Could you check a few things on this model? Use its own coordinates, in mm. Face numbers are marked on the shaded views. A direction names the side the tool comes from. Coordinates: 2 decimals unless noted, no trailing zeros. Loops run counter-clockwise (first coordinate to the right, second up) from the corner with the lowest first, then second, coordinate; pieces in that order, holes last.
Autodesk Inventor part; units mm, degrees
ref_plane "YZ Plane" through (0, 0, 0) normal (1, 0, 0) x (0, 1, 0)
ref_plane "XZ Plane" through (0, 0, 0) normal (0, 1, 0) x (-1, 0, 0)
ref_plane "XY Plane" through (0, 0, 0) normal (0, 0, 1) x (1, 0, 0)
sketch "Sketch1" plane through (0, 0, 0) normal (0, 1, 0) x (-1, 0, 0)
  line L0 (-21, -21) -> (21, -21)
  line L1 (21, -21) -> (21, 21)
  line L2 (21, 21) -> (-21, 21)
  line L3 (-21, 21) -> (-21, -21)
  line L4 (-21, -21) -> (21, 21) construction
  line L5 (21, -21) -> (-21, 21) construction
  point P0 (0, 0)
  dimension "d0" = 42
  dimension "d1" = 42
extrude "Extrusion1" add sketch "Sketch1" along normal blind 9
chamfer "Chamfer1" distance 6 angle 45 4 edges at (21, 4.5, -21) (-21, 4.5, -21) (-21, 4.5, 21) (21, 4.5, 21)
sketch "Sketch2" plane through (0, 9, 0) normal (0, 1, 0) x (1, 0, 0)
  point P0 (0, 0)
sketch "Sketch3" plane through (0, 0, 0) normal (0, -1, 0) x (1, 0, 0)
  circle A0 centre (0, 0) radius 5
  dimension "d7" = 10
extrude "Extrusion2" cut sketch "Sketch3" against normal up to surface (9 mm away)
sketch "Sketch4" plane through (0, 9, 0) normal (0, 1, 0) x (1, 0, 0)
  circle A0 centre (-15.5, -15.5) radius 1.5
  line L0 (-15, -21) -> (15, -21)
  line L1 (-21, 15) -> (-21, -15)
  point P0 (0, 0)
  dimension "d10" = 3
  dimension "d11" = 5.5
  dimension "d12" = 5.5
extrude "Extrusion3" cut sketch "Sketch4" against normal up to surface (9 mm away)
mirror "Mirror1" about plane through (0, 0, 0) normal (1, 0, 0) of "Extrusion3"
mirror "Mirror2" about plane through (0, 0, 0) normal (0, 0, 1) of "Extrusion3", "Mirror1"
sketch "Sketch6" plane through (0, 0, 0) normal (0, -1, 0) x (1, 0, 0)
  circle A0 centre (15.5, -15.5) radius 1.5
  circle A1 centre (-15.5, -15.5) radius 1.5
  circle A2 centre (15.5, 15.5) radius 1.5
  circle A3 centre (-15.5, 15.5) radius 1.5
  circle A4 centre (0, 0) radius 5
  line L0 (15, 21) -> (21, 15)
  line L1 (-15, 21) -> (15, 21)
  line L2 (-21, 15) -> (-15, 21)
  line L3 (-21, -15) -> (-21, 15)
  line L4 (-15, -21) -> (-21, -15)
  line L5 (15, -21) -> (-15, -21)
  line L6 (21, -15) -> (15, -21)
  line L7 (21, 15) -> (21, -15)
  line L8 (8, -21) -> (-8, -21)
  line L9 (-8, -21) -> (-8, -25)
  line L10 (-8, -25) -> (8, -25)
  line L11 (8, -25) -> (8, -21)
  dimension "d20" = 16
  dimension "d21" = 8
  dimension "d24" = 4
extrude "Extrusion5" add sketch "Sketch6" against normal blind 4 contours L11 L10 L9 L5
fillet "Fillet1" radius 0.5 2 edges at (8, 2, -25) (-8, 2, -25)
sketch "Sketch7" plane through (15, 9, -21) normal (0, 0, -1) x (-1, 0, 0)
  line L0 (23, -5) -> (23, -9)
  line L1 (23, -9) -> (30, -9)
  line L2 (30, 0) -> (30, -9)
  line L3 (0, 0) -> (30, 0)
  line L4 (0, -9) -> (0, 0)
  line L5 (0, -9) -> (7, -9)
  line L6 (7, -9) -> (7, -5)
  line L7 (7, -5) -> (23, -5)
  line L8 (7, -5) -> (23, -5)
  line L9 (23, -5) -> (23, 0)
  line L10 (23, 0) -> (7, 0)
  line L11 (7, 0) -> (7, -5)
  point P0 (15, -9)
extrude "Extrusion6" cut sketch "Sketch7" against normal blind 10 contours L7 L11 L3 L9
sketch "Sketch8" plane through (15, 9, -11) normal (0, 0, -1) x (-1, 0, 0)
  line L0 (23, -5) -> (7, -5)
  line L1 (23, 0) -> (23, -5)
  line L2 (7, 0) -> (23, 0)
  line L3 (7, -5) -> (7, 0)
  line L4 (23, 0) -> (23, -5)
  line L5 (7, -4.3) -> (23, -4.3)
  line L6 (23, -4.3) -> (23, -4.8)
  line L7 (23, -4.8) -> (7, -4.8)
  line L8 (7, -4.8) -> (7, -4.3)
  point P0 (15, -9)
  dimension "d28" = 0.5
  dimension "d29" = 0.2
extrude "Extrusion7" add sketch "Sketch8" along normal blind 15 contours L7 L3 L5 L1
sketch "Sketch9" plane through (15, 9, -11) normal (0, 0, -1) x (-1, 0, 0)
  point P0 (15, -9)
sketch "Sketch10" plane through (0, 0, 0) normal (0, -1, 0) x (1, 0, 0)
  circle A0 centre (15.5, 15.5) radius 1.5
  circle A1 centre (15.5, 15.5) radius 3
  point P0 (0, 0)
  dimension "d32" = 6
extrude "Extrusion8" cut sketch "Sketch10" against normal blind 3
mirror "Mirror3" about plane through (0, 0, 0) normal (1, 0, 0) of "Extrusion8"
mirror "Mirror4" about plane through (0, 0, 0) normal (0, 0, 1) of "Extrusion8", "Mirror3"
equation "\"d12\" = d11"
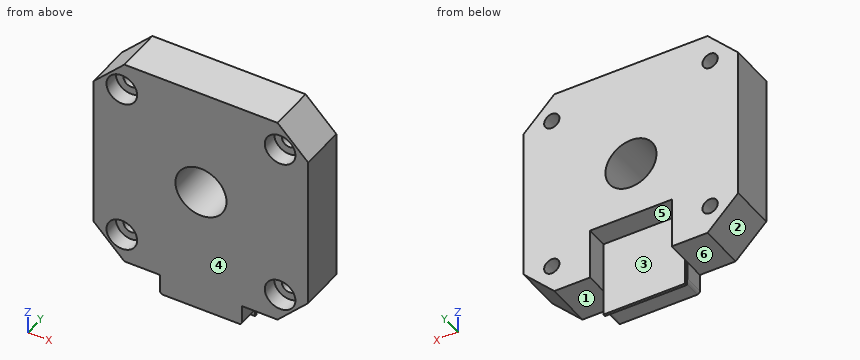
(1) Imagine slicing it at B-B, the plane x = 0. Write out the boundary of the cut face in (y, z).
Answers:
outline: (0, -25) - (4, -25) - (4, -11) - (4.2, -11) - (4.2, -26) - (4.7, -26) - (4.7, -11) - (9, -11) - (9, -5) - (0, -5) - close; (0, 5) - (9, 5) - (9, 21) - (0, 21) - close
(2) Imagine slicing it at A-A, the plane z = 0. Write out the boundary of the cut face in (x, y).
Answers:
outline: (-21, 0) - (-5, 0) - (-5, 9) - (-21, 9) - close; (5, 0) - (21, 0) - (21, 9) - (5, 9) - close
(3) Imagine slicing it at C-C, the plane y = 1. Write out the boundary of the cut face in (x, z), and give its area (3 significant figures).
Answers:
outline: (-21, -15) - (-15, -21) - (-8, -21) - (-8, -24.5) arc R0.5 ccw to (-7.5, -25) - (7.5, -25) arc R0.5 ccw to (8, -24.5) - (8, -21) - (15, -21) - (21, -15) - (21, 15) - (15, 21) - (-15, 21) - (-21, 15) - close; hole circle Ø6 at (-15.5, -15.5); hole circle Ø6 at (-15.5, 15.5); hole circle Ø10 at (0, 0); hole circle Ø6 at (15.5, -15.5); hole circle Ø6 at (15.5, 15.5)
area: 1,560 mm2
(4) Which directions (+Z, -Z, +X, -X, +Y, -Y) give clear straight access to the entire face, cutting with the end or side of a thin tool? Please do the marked faces 4, 5 and 6.
Answers:
face 4: +Z, -Z, +X, -X, -Y
face 5: -Z, +Y
face 6: -Z, -X, +Y, -Y
(5) For pin 1 (1.8 mm diameter, centred on x = -14.5, z = 14, fed in from -Y); pin 2 (0.6 mm diameter, centred on y = 4.5, z = -22.5, fed in from +X); pin 3 (1 mm diameter, centred on y = 1.5, z = 16.5, fed in from +X), each with a flat end and sliding along its axis, tell me the tip position at first contact or that it passes through.
Answers:
pin 1: stops at y = 3
pin 2: stops at x = 8
pin 3: stops at x = 20
(6) We'd pull the mould along X, two halves only. Please class the marked faces 1, 2 and 3: +X half, -X half, draft (parallel to the pull), parting line (faces both ways), or undercut.
Answers:
face 1: draft
face 2: -X half
face 3: undercut
(7) I need wall thicknesses on probe 1 along Z at (x, y) = (-16.5, 0.5); probe 2 along X at (y, z) = (5.9, 15.5); probe 3 along X at (y, z) = (7, -13). Which ranges of each line are inside material? Lowest first, please.
Answers:
probe 1: z = -19.5 to -18.33, -12.67 to 12.67, 18.33 to 19.5
probe 2: x = -20.5 to -17, -14 to 14, 17 to 20.5
probe 3: x = -21 to -8, 8 to 21
(8) Imagine slicing it at D-D, the plane x = -16. Write out the boundary of the cut face in (y, z).
Answers:
outline: (0, -20) - (9, -20) - (9, -16.91) - (3, -16.91) - (3, -18.46) - (0, -18.46) - close; (0, -12.54) - (3, -12.54) - (3, -14.09) - (9, -14.09) - (9, 14.09) - (3, 14.09) - (3, 12.54) - (0, 12.54) - close; (0, 18.46) - (3, 18.46) - (3, 16.91) - (9, 16.91) - (9, 20) - (0, 20) - close
